Geometry: final body of the model. Coordinates: model frame, mm. Give positions to 0.01 mm unless a question says otherwise; leave off trailing zeros. Order: outer loops, then holes, each group sorted by start corner. A loop starts at its lowest first (then second) coordinate and runs counter-clockwise, first axis right, second up. Notation, with made-up numbers: (74.5, 73) - (105.5, 73) arc R27 cw to (105.5, 92) - close; hole circle Ø11 at (5.25, 49.5). An arc over 180 degrees is marked (long way). Use one line per item in the form item = value.
from build123d import *

# Parameters (mm, degrees)
SKETCH1_W           = 78.232
SKETCH1_H           = 218.44
BOSS_EXTRUDE1_DEPTH = 1.4605
SKETCH2_W           = 2.921
SKETCH2_H           = 25.4
SKETCH2_H_2         = 12.7
CUT_EXTRUDE1_DEPTH  = 2.921
SKETCH3_W           = 6.35
SKETCH3_H           = 2.921
BOSS_EXTRUDE2_DEPTH = 6.0452
SKETCH5_W           = 6.35
SKETCH5_H           = 160.02
CUT_EXTRUDE2_DEPTH  = 122.756560513


with BuildPart() as part:
    # Sketch1 → Boss-Extrude1 (new, symmetric)
    with BuildSketch(Plane.XY):
        Rectangle(SKETCH1_W, SKETCH1_H)
    extrude(amount=BOSS_EXTRUDE1_DEPTH, both=True)

    # Sketch2 → Cut-Extrude1 (cut)
    with BuildSketch(Plane.XY.offset(1.4605)):
        with Locations((-37.6555, -96.52)):
            Rectangle(SKETCH2_W, SKETCH2_H)
        with Locations((-37.6555, -45.72)):
            Rectangle(SKETCH2_W, SKETCH2_H)
        with Locations((-37.6555, 5.08)):
            Rectangle(SKETCH2_W, SKETCH2_H)
        with Locations((-37.6555, 49.53)):
            Rectangle(SKETCH2_W, SKETCH2_H_2)
        with Locations((37.6555, 49.53)):
            Rectangle(SKETCH2_W, SKETCH2_H_2)
        with Locations((37.6555, 5.08)):
            Rectangle(SKETCH2_W, SKETCH2_H)
        with Locations((37.6555, -96.52)):
            Rectangle(SKETCH2_W, SKETCH2_H)
        with Locations((37.6555, -45.72)):
            Rectangle(SKETCH2_W, SKETCH2_H)
    extrude(amount=-CUT_EXTRUDE1_DEPTH, mode=Mode.SUBTRACT)

    # Sketch3 → Boss-Extrude2 (add)
    with BuildSketch(Plane(origin=(0, 109.22, 0), x_dir=(1, 0, 0), z_dir=(0, 1, 0))):
        with Locations((31.75, 0)):
            Rectangle(SKETCH3_W, SKETCH3_H)
        with Locations((19.05, 0)):
            Rectangle(SKETCH3_W, SKETCH3_H)
        with Locations((6.35, 0)):
            Rectangle(SKETCH3_W, SKETCH3_H)
        with Locations((-6.35, 0)):
            Rectangle(SKETCH3_W, SKETCH3_H)
        with Locations((-19.05, 0)):
            Rectangle(SKETCH3_W, SKETCH3_H)
        with Locations((-31.75, 0)):
            Rectangle(SKETCH3_W, SKETCH3_H)
    extrude(amount=BOSS_EXTRUDE2_DEPTH)

    # Sketch5 → Cut-Extrude2 (cut, through all)
    with BuildSketch(Plane.XY.offset(1.4605)):
        with Locations((-12.7, -22.86)):
            Rectangle(SKETCH5_W, SKETCH5_H)
        with Locations((12.7, -22.86)):
            Rectangle(SKETCH5_W, SKETCH5_H)
    extrude(amount=-CUT_EXTRUDE2_DEPTH, mode=Mode.SUBTRACT)


solid = part.part
(1) Cut plane B-B on x = -26. Output: boundary loops of the cut face in (y, z), plus the area to 3 significant figures.
Computed values:
outline = (-109.22, -1.46) - (109.22, -1.46) - (109.22, 1.46) - (-109.22, 1.46) - close
area = 638 mm²
(2) Contact query for flat-ended pins moving along their axis: pin 1 Ø1.5 at (x, z) = (13, 0) entering from +Y; pin 2 Ø1.5 at (y, z) = (112, 0.5) entering from -X (3 decimals); pin 3 Ø1.5 at (y, z) = (50.5, 0) entering from -X (3 decimals). Output: stop coordinate, or through.
Computed values:
pin_1 = 109.22
pin_2 = -34.925
pin_3 = -36.195
(3) Cut plane C-C on z = 0.1. Give the number of separate pieces and of enclosed holes in the cut face, plus the area to 3 significant figures.
Computed values:
separate_pieces = 1
enclosed_holes = 2
area = 14,800 mm²
(4) Cut plane A-A on y = 10.5. Output: boundary loops of the cut face in (x, z) (1 decimal), plus the area to 3 significant figures.
Computed values:
outline = (-36.2, -1.5) - (-15.9, -1.5) - (-15.9, 1.5) - (-36.2, 1.5) - close; (-9.5, -1.5) - (9.5, -1.5) - (9.5, 1.5) - (-9.5, 1.5) - close; (15.9, -1.5) - (36.2, -1.5) - (36.2, 1.5) - (15.9, 1.5) - close
area = 174 mm²
(5) Ray query, line 1 along X through (y, z) = (-11, -1.1) (3 decimals); line 2 along X through (y, z) = (-46, -0.4) (3 decimals); line 3 along Y through (x, z) = (12.5, 0.1). Return the intervals inside material, ascending.
Computed values:
line_1 = -39.116 to -15.875, -9.525 to 9.525, 15.875 to 39.116
line_2 = -36.195 to -15.875, -9.525 to 9.525, 15.875 to 36.195
line_3 = -109.22 to -102.87, 57.15 to 109.22
